```python
from build123d import *

# Parameters (mm, degrees)
SKETCH1_W               = 100
SKETCH1_H               = 100
BOSS_EXTRUDE1_DEPTH     = 300
SHELL1_T                = -5
SKETCH5_W               = 29.520338389
SKETCH5_H               = 280
SKETCH5_W_2             = 30.177604706
CUT_EXTRUDE3_DEPTH      = 332.662479036
CUT_EXTRUDE4_DEPTH      = 332.662479036
CUT_EXTRUDE4_DEPTH_BACK = 332.662479036
SKETCH7_W               = 22.211506019
SKETCH7_H               = 280
SKETCH7_W_2             = 24.857728264
SKETCH8_R               = 2.210472055
BOSS_EXTRUDE2_DEPTH     = 1
BOSS_EXTRUDE3_DEPTH     = 2
SKETCH10_R              = 1
BOSS_EXTRUDE4_DEPTH     = 2


with BuildPart() as part:
    # Sketch1 → Boss-Extrude1 (new body)
    with BuildSketch(Plane(origin=(0, 0, 0), x_dir=(1, 0, 0), z_dir=(0, 1, 0))):
        with Locations((50, 50)):
            Rectangle(SKETCH1_W, SKETCH1_H)
    extrude(amount=BOSS_EXTRUDE1_DEPTH)

    # Shell1
    shell1_openings = [part.faces().sort_by_distance(p)[0] for p in [
        (50, 300, -50),
    ]]
    offset(amount=SHELL1_T, openings=shell1_openings, kind=Kind.INTERSECTION)

    # Sketch5 → Cut-Extrude3 (cut, through all)
    with BuildSketch(Plane(origin=(100, 0, 0), x_dir=(0, 0, -1), z_dir=(1, 0, 0))):
        with Locations((24.760169195, 150)):
            Rectangle(SKETCH5_W, SKETCH5_H)
        with Locations((74.911197647, 150)):
            Rectangle(SKETCH5_W_2, SKETCH5_H)
    extrude(amount=-CUT_EXTRUDE3_DEPTH, mode=Mode.SUBTRACT)

    # Sketch7 → Cut-Extrude4 (cut, two sides: drawn at the far end of the back side and taken through both)
    with BuildSketch(Plane(origin=(0, 0, -100), x_dir=(-1, 0, 0), z_dir=(0, 0, -1)).offset(-CUT_EXTRUDE4_DEPTH_BACK)):
        with Locations((-78.89424699, 150)):
            Rectangle(SKETCH7_W, SKETCH7_H)
        with Locations((-22.428864132, 150)):
            Rectangle(SKETCH7_W_2, SKETCH7_H)
    extrude(amount=CUT_EXTRUDE4_DEPTH + CUT_EXTRUDE4_DEPTH_BACK, mode=Mode.SUBTRACT)

    # Sketch8 → Boss-Extrude2 (add)
    with BuildSketch(Plane(origin=(0, 0, -5), x_dir=(-1, 0, 0), z_dir=(0, 0, -1))):
        with Locations((-52.421904505, 126.432189468)):
            Circle(SKETCH8_R)
    extrude(amount=BOSS_EXTRUDE2_DEPTH)

    # Sketch9 → Boss-Extrude3 (add)
    with BuildSketch(Plane(origin=(0, 5, 0), x_dir=(1, 0, 0), z_dir=(0, 1, 0))):
        with BuildLine():
            ThreePointArc((51, 50), (50, 51), (49, 50))
            Line((49, 50), (51, 50))
        make_face()
        with BuildLine():
            Line((51, 50), (49, 50))
            ThreePointArc((49, 50), (50, 49), (51, 50))
        make_face()
    extrude(amount=BOSS_EXTRUDE3_DEPTH)

    # Sketch10 → Boss-Extrude4 (add)
    with BuildSketch(Plane.ZY.offset(-95)):
        with Locations((-50.457978823, 101.351671268)):
            Circle(SKETCH10_R)
    extrude(amount=BOSS_EXTRUDE4_DEPTH)


solid = part.part
```
The model under review builds one solid part; all positions refer to its coordinate system, in mm. A direction names the side the tool comes from. Give positions to 0.01 mm unless a question says otherwise; leave off trailing zeros. Write each loop counter-clockwise with the first axis right and the second up, starting at its lowest first coordinate (ties: lowest second). Pieces come first, ordered by that corner, then holes. Notation, with made-up numbers: (-6.75, -8) -> (23.25, -8) arc R20 ccw to (23.25, 4) -> close; hole circle Ø9 at (48, 63.5). An arc over 180 degrees is marked (long way). Answer in a Markdown table with one row per item.
1) Add section A-A on x = 27.5. State the section outline as (y, z) points.
Worked answers:
| item | result |
|---|---|
| outline | (0, -100) -> (10, -100) -> (10, -95) -> (5, -95) -> (5, -5) -> (10, -5) -> (10, 0) -> (0, 0) -> close; (290, -100) -> (300, -100) -> (300, -95) -> (290, -95) -> close; (290, -5) -> (300, -5) -> (300, 0) -> (290, 0) -> close |
2) For L1, parallel to X at y = 88, z = -4.5; L2, parallel to Z at x = 96, y = 215.5; L3, parallel to Z at x = 8, y = 93.5, list the stretches that pass through material, from the lowest coordinate up. Write a range as [from, to].
Worked answers:
| item | result |
|---|---|
| L1 | [0, 10], [34.86, 67.79], [90, 100] |
| L2 | [-100, -90], [-59.82, -39.52], [-10, 0] |
| L3 | [-100, -95], [-5, 0] |
3) Mouldability with a two-part tool opening along X and no side actions: class faces 4 (the flat face through (95, 163, -46)), 5 (the flat face through (0, 149, -53)), 6 (the flat face through (98, 290, -75)) as +X half, -X half, draft (parallel to the pull), parting line (faces both ways), or undercut.
Worked answers:
| item | result |
|---|---|
| face 4 | undercut |
| face 5 | -X half |
| face 6 | draft |
4) Clearance check with flat-ended pins moving along their axes: P1, Ø8, axis at x = 69.5, z = -46, coming from the +Y side; P2, Ø2, axis at x = 50, z = -50.5, coming from the +Y side. State where each tip first meets the part, or that it passes through.
Worked answers:
| item | result |
|---|---|
| P1 | y = 5 |
| P2 | y = 7 |
5) Tool access review of faces 1 (the flat face through (39, 150, -95)), 2 (the flat face through (3, 148, -10)), 3 (the flat face through (23, 10, -97)): name each direction out of +Z, -Z, +X, -X, +Y, -Y from which nothing blocks a thin tool from reaching the whole face with its end or side.
Worked answers:
| item | result |
|---|---|
| face 1 | +Y |
| face 2 | +X, -X |
| face 3 | +Z, -Z |
6) Add section C-C on x = 40. State the section outline as (y, z) points, plus the area to 3 significant figures.
Worked answers:
| item | result |
|---|---|
| outline | (0, -100) -> (300, -100) -> (300, -95) -> (5, -95) -> (5, -5) -> (300, -5) -> (300, 0) -> (0, 0) -> close |
| area | 3,450 mm² |
7) Add section D-D on y = 209. Count the separate pieces of the cut face and the enclosed holes in it, plus the area to 3 significant figures.
Worked answers:
| item | result |
|---|---|
| separate pieces | 8 |
| enclosed holes | 0 |
| area | 832 mm² |
8) Add section B-B on z = -17.5. State the section outline as (x, y) points, plus the area to 3 significant figures.
Worked answers:
| item | result |
|---|---|
| outline | (0, 0) -> (100, 0) -> (100, 10) -> (95, 10) -> (95, 5) -> (5, 5) -> (5, 10) -> (0, 10) -> close; (0, 290) -> (5, 290) -> (5, 300) -> (0, 300) -> close; (95, 290) -> (100, 290) -> (100, 300) -> (95, 300) -> close |
| area | 650 mm² |
